Design review of the part built by this model. Coordinates are the model's own, in mm. Coordinates: 2 decimals unless noted, no trailing zeros. Write each loop counter-clockwise with the first axis right and the second up, starting at its lowest first coordinate (ties: lowest second). Pieces come first, ordered by that corner, then holes. Notation, with made-up numbers: (-32, 31) -> (-7, 31) arc R20 ccw to (-7, 59) -> close; hole circle Ø6 at (28.25, -33). An arc over 180 degrees is marked (long way). Answer in a Markdown table with one row per item. Add a question column.
Item 1: Take a section at C-C, the plane y = -0.7. Write out the cut boundary in (x, z).
Item 2: Take a section at A-A, the plane x = -11. Write out the cut boundary in (y, z).
Item 3: Take a section at B-B, the plane z = 33. Write out the cut boundary in (x, y).
Item 4: Take a section at D-D, the plane z = 7. Write out the cut boundary in (x, y), and give its area (3 significant figures).
Item 5: To check wall thickness, follow line 1 (Z direction, x = -5.5, y = -2.3); line 2 (Z direction, x = 5.25, y = -0.8); line 3 (Z direction, x = 7.25, y = -2). State the ranges of each line that lie inside material, in increasing order.
Item 6: Clearance check with a flat-ended pin moving along its axis: P1, Ø0.8, axis at y = -1.5, z = 17.5, coming from the +X side. State where the tip first meets the part, or that it passes through.
from build123d import *

# Parameters (mm, degrees)
F1_DEPTH = 2.54
F2_R     = 1.589484
F3_DEPTH = 2.54


with BuildPart() as f1:
    # F0 (on Front) → F1 (new body)
    with BuildSketch(Plane.XZ):
        Polygon((-12.964887, 6.35), (-12.964887, 0), (9.895113, 0), (9.895113, 6.35), (3.112477, 6.35), (3.112477, 29.21), (9.895113, 29.21), (9.895113, 35.56), (-12.964887, 35.56), (-12.964887, 29.21), (-4.926205, 29.21), (-4.926205, 6.35), align=None)
    extrude(amount=F1_DEPTH)

    # F2 (on face) → F3 (cut)
    with BuildSketch(Plane.XZ.offset(2.54)):
        with Locations((6.503795, 32.47159)):
            Circle(F2_R)
    extrude(amount=-F3_DEPTH, mode=Mode.SUBTRACT)


solid = f1.part
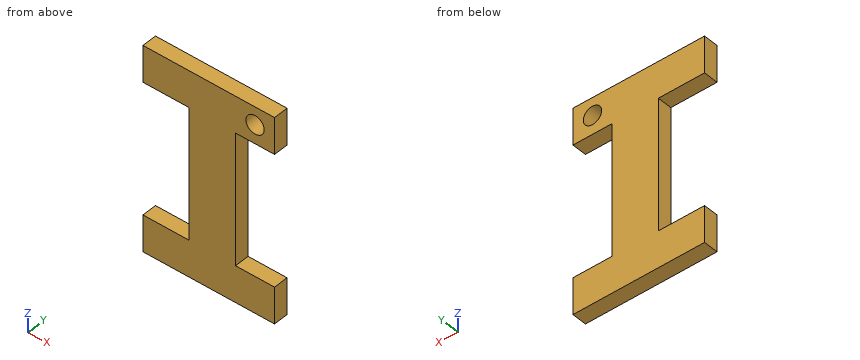
Answers:
| question | item | result |
|---|---|---|
| 1 | outline | (-12.96, 0) -> (9.9, 0) -> (9.9, 6.35) -> (3.11, 6.35) -> (3.11, 29.21) -> (9.9, 29.21) -> (9.9, 35.56) -> (-12.96, 35.56) -> (-12.96, 29.21) -> (-4.93, 29.21) -> (-4.93, 6.35) -> (-12.96, 6.35) -> close; hole circle Ø3.18 at (6.5, 32.47) |
| 2 | outline | (-2.54, 0) -> (0, 0) -> (0, 6.35) -> (-2.54, 6.35) -> close; (-2.54, 29.21) -> (0, 29.21) -> (0, 35.56) -> (-2.54, 35.56) -> close |
| 3 | outline | (-12.96, -2.54) -> (5, -2.54) -> (5, 0) -> (-12.96, 0) -> close; (8, -2.54) -> (9.9, -2.54) -> (9.9, 0) -> (8, 0) -> close |
| 4 | outline | (-4.93, -2.54) -> (3.11, -2.54) -> (3.11, 0) -> (-4.93, 0) -> close |
| 4 | area | 20.4 mm^2 |
| 5 | line 1 | z = 0 to 6.35, 29.21 to 35.56 |
| 5 | line 2 | z = 0 to 6.35, 29.21 to 31.49, 33.45 to 35.56 |
| 5 | line 3 | z = 0 to 6.35, 29.21 to 31.07, 33.88 to 35.56 |
| 6 | P1 | stops at x = 3.11 |
